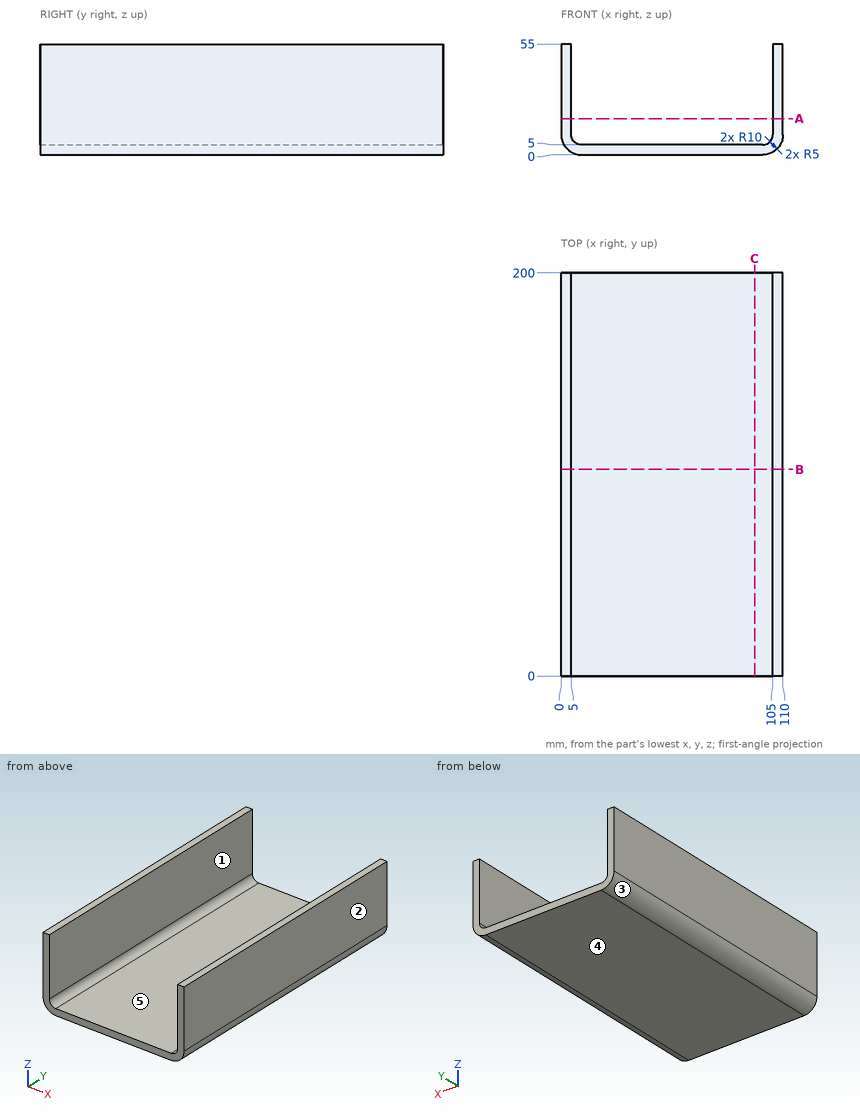
The figure shows three views and two pictorial views of one solid part (mm, origin at its lowest corner). Answer the questions. A direction names the side the tool comes from. Give positions to 0.01 mm unless a question says otherwise; leave off trailing zeros. Loops run counter-clockwise (first coordinate to the right, second up) from the corner with the lowest first, then second, coordinate; pieces in that order, holes last. Notation, with made-up numbers: (55, 40) -> (106, 40) arc R18 cw to (106, 49) -> close; hole circle Ø5 at (10, 44). An arc over 180 degrees is marked (long way). Use a Markdown table: item, result. Add a question column.
1. Section A-A on z = 18 is taken. Determine the outline of the cut face in (x, y), and give its area (3 significant figures).
2. Section B-B on y = 102.5 is taken. Determine the outline of the cut face in (x, z), and give its area (3 significant figures).
3. Find the intervals of material crossed by probe 1 along X at (y, z) = (100, 28.5); probe 2 along Z at (x, y) = (81, 48.5); probe 3 along X at (y, z) = (80, 6), in increasing order.
4. Determine the mould class of the marked faces 1, 2 and 3 for opening direction X: released by +X, released by -X, zero draft, split by the parting line, or undercut.
5. Flat-ended cylindrical pins translate along their axes: pin 1 Ø1 at (y, z) = (161, 5.5) entering from +X; pin 2 Ø4 at (x, y) = (92.5, 117.5) entering from +Z. Find the tip coordinate at first contact, or state that the pin passes through.
6. Section C-C on x = 96 is taken. Determine the outline of the cut face in (y, z).
7. For the marked faces 4 and 5, determine the directions among +Z, -Z, +X, -X, +Y, -Y from which every point of the face is accessible in a straight line to the end or side of a thin tool.
Results below:
| question | item | result |
|---|---|---|
| 1 | outline | (0, 0) -> (5, 0) -> (5, 200) -> (0, 200) -> close; (105, 0) -> (110, 0) -> (110, 200) -> (105, 200) -> close |
| 1 | area | 2,000 mm^2 |
| 2 | outline | (0, 10) arc R10 ccw to (10, 0) -> (100, 0) arc R10 ccw to (110, 10) -> (110, 55) -> (105, 55) -> (105, 10) arc R5 cw to (100, 5) -> (10, 5) arc R5 cw to (5, 10) -> (5, 55) -> (0, 55) -> close |
| 2 | area | 1,020 mm^2 |
| 3 | probe 1 | x = 0 to 5, 105 to 110 |
| 3 | probe 2 | z = 0 to 5 |
| 3 | probe 3 | x = 0.83 to 7, 103 to 109.17 |
| 4 | face 1 | undercut |
| 4 | face 2 | released by +X |
| 4 | face 3 | released by -X |
| 5 | pin 1 | stops at x = 109.17 |
| 5 | pin 2 | stops at z = 5 |
| 6 | outline | (0, 0) -> (200, 0) -> (200, 5) -> (0, 5) -> close |
| 7 | face 4 | -Z, +X, -X, +Y, -Y |
| 7 | face 5 | +Z, +Y, -Y |
